Could you check a few things on this model? Use its own coordinates, in mm. A direction names the side the tool comes from. Give positions to 0.01 mm unless a question says otherwise; leave off trailing zeros. Loops run counter-clockwise (first coordinate to the right, second up) from the corner with the lowest first, then second, coordinate; pieces in that order, holes last. Notation, with made-up numbers: (-17, -21.75) -> (40, -21.75) arc R23 cw to (40, 0.25) -> close; hole circle Ø3 at (33.25, -30). An arc over 180 degrees is marked (long way). Write each question's results on one line, items separated by ' | '. Start each with the question number.
Q1. We'd pull the mould along Z, two halves only. Please class faces 4 (the face through (803.656, -20, -14)), 5 (the face through (802.4, 12.16, -23.38)), 6 (the face through (553.212, -5.162, -23.246)): released by +Z, released by -Z, zero draft, split by the parting line, or undercut.
Q2. If I drill on line 1 along Y through (x, z) = (14, 0); line 2 along Y through (x, z) = (435, -2.5), over which ranges is the centre line in solid material (lowest first)?
Q3. Which directions (+Z, -Z, +X, -X, +Y, -Y) give clear straight access to the entire face, cutting with the end or side of a thin tool? Please do faces 1 (the face through (295.656, 0, 0)), 2 (the face through (788.416, -15, 35)), 3 (the face through (794.855, 37.855, -11.921)).
Q4. If we section it at A-A, the plane x = 672: List the corners of the cut face in (y, z) for me (1 decimal), plus the area to 3 significant figures.
Q5. If we section it at B-B, the plane x = 194: List the corners of the cut face in (y, z) for me.
Q6. Will these pins go through, and if not, where does the flat tip stop? P1, Ø12, axis at x = 344, z = -24, coming from the +Y side; P2, Ø4, axis at x = 256.5, z = -19, coming from the +Y side; P3, Ø8, axis at x = 384, y = -11, coming from the +Z side; P4, Ø22.5, axis at y = -16, z = -12, coming from the -X side.
from build123d import *

# Parameters (mm, degrees)
CHAMFER1_SIZE                                       = 2.54
CSK_FOR_3_8_FLAT_HEAD_MACHINE_SCREW_100_D           = 10.0838
CSK_FOR_3_8_FLAT_HEAD_MACHINE_SCREW_100_DEPTH       = 25.4
CSK_FOR_3_8_FLAT_HEAD_MACHINE_SCREW_100_CSINK_D     = 19.3548
CSK_FOR_3_8_FLAT_HEAD_MACHINE_SCREW_100_CSINK_ANGLE = 100
CSK_FOR_3_8_FLAT_HEAD_MACHINE_SCREW_100_TIP         = 3.029479155
FILLET2_R                                           = 1.27
BOSS_EXTRUDE1_START                                 = 2.54
SKETCH5_R                                           = 26.3525
SKETCH5_R_2                                         = 23.8125
BOSS_EXTRUDE1_DEPTH                                 = 2.54
SKETCH6_R                                           = 23.8125
CUT_EXTRUDE1_DEPTH                                  = 508


with BuildPart() as part:
    # Sketch1 → Revolve1 (revolve)
    with BuildSketch(Plane.XY):
        Polygon((0, 0), (0, 12.7), (25.4, 12.7), (25.4, 23.8125), (44.45, 23.8125), (44.45, 37.6555), (788.416, 37.6555), (788.416, 39.6875), (801.116, 39.6875), (801.116, 0), align=None)
    revolve(axis=Axis((801.116, 0, 0), (-1, 0, 0)))

    # Chamfer1
    chamfer1_edges = [part.edges().sort_by_distance(p)[0] for p in [
        (25.4, -23.8125, 0),
    ]]
    chamfer(chamfer1_edges, length=CHAMFER1_SIZE)

    # CSK for 3/8 Flat Head Machine Screw (100)1
    with Locations(Plane.ZY):
        with Locations((0, 0)):
            CounterSinkHole(CSK_FOR_3_8_FLAT_HEAD_MACHINE_SCREW_100_D / 2, CSK_FOR_3_8_FLAT_HEAD_MACHINE_SCREW_100_CSINK_D / 2, depth=CSK_FOR_3_8_FLAT_HEAD_MACHINE_SCREW_100_DEPTH, counter_sink_angle=CSK_FOR_3_8_FLAT_HEAD_MACHINE_SCREW_100_CSINK_ANGLE)
            with Locations((0, 0, -(CSK_FOR_3_8_FLAT_HEAD_MACHINE_SCREW_100_DEPTH + CSK_FOR_3_8_FLAT_HEAD_MACHINE_SCREW_100_TIP / 2))):  # 118° drill point
                Cone(0, CSK_FOR_3_8_FLAT_HEAD_MACHINE_SCREW_100_D / 2, CSK_FOR_3_8_FLAT_HEAD_MACHINE_SCREW_100_TIP, mode=Mode.SUBTRACT)

    # Fillet2
    fillet2_edges = [part.edges().sort_by_distance(p)[0] for p in [
        (0, -12.7, 0),
    ]]
    fillet(fillet2_edges, radius=FILLET2_R)

    # Sketch5 → Boss-Extrude1 (add)
    with BuildSketch(Plane(origin=(801.116, 0, 0), x_dir=(0, 0, -1), z_dir=(1, 0, 0)).offset(BOSS_EXTRUDE1_START)):
        with Locations(Location((0, 0, 0), (0, 0, 90))):
            Circle(SKETCH5_R)
        with Locations(Location((0, 0, 0), (0, 0, 90))):
            Circle(SKETCH5_R_2, mode=Mode.SUBTRACT)
    extrude(amount=-BOSS_EXTRUDE1_DEPTH)

    # Sketch6 → Cut-Extrude1 (cut)
    with BuildSketch(Plane(origin=(803.656, 0, 0), x_dir=(0, 0, -1), z_dir=(1, 0, 0))):
        with Locations(Location((0, 0, 0), (0, 0, 90))):
            Circle(SKETCH6_R)
    extrude(amount=-CUT_EXTRUDE1_DEPTH, mode=Mode.SUBTRACT)


solid = part.part
Final values:
1) face 4: zero draft | face 5: split by the parting line | face 6: undercut
2) line 1: y = -12.7 to -5.04, 5.04 to 12.7 | line 2: y = -37.57 to -23.68, 23.68 to 37.57
3) face 1: +X | face 2: -X | face 3: +X, -X
4) outline: circle Ø75.3 at (0, 0); hole circle Ø47.6 at (0, 0) | area: 2,670 mm²
5) outline: circle Ø75.31 at (0, 0)
6) P1: stops at y = 33.07 | P2: stops at y = 33.6 | P3: stops at z = 37 | P4: stops at x = 0
